from build123d import *

# Parameters (mm, degrees)
SKETCH_1_W                   = 110
SKETCH_1_H                   = 110
EXTRUDE_1_DEPTH              = 110
SKETCH_2_W                   = 100
SKETCH_2_H                   = 100
CUT_EXTRUDE_1_DEPTH          = 105
SKETCH_3_W                   = 13.484754144
SKETCH_3_H                   = 100
CUT_EXTRUDE_2_DEPTH          = 105
HOLE_WIZARD_M4_6_D           = 3.3
HOLE_WIZARD_M4_6_CSINK_D     = 4.05
HOLE_WIZARD_M4_6_CSINK_ANGLE = 90
HOLE_WIZARD_M4_7_D           = 3.3
HOLE_WIZARD_M4_7_CSINK_D     = 4.05
HOLE_WIZARD_M4_7_CSINK_ANGLE = 90
PATTERN_CIRCULAR_2_COUNT     = 6


# Read off the part's stored shape, not the designer's step: 阵列(圆周)1
with BuildPart() as part:
    # 草图1 → 凸台-拉伸1 (new body)
    with BuildSketch(Plane(origin=(0, 0, 0), x_dir=(1, 0, 0), z_dir=(0, 1, 0))):
        Rectangle(SKETCH_1_W, SKETCH_1_H)
    extrude(amount=EXTRUDE_1_DEPTH)

    # 草图2 → 切除-拉伸1 (cut)
    with BuildSketch(Plane(origin=(0, 110, 0), x_dir=(1, 0, 0), z_dir=(0, 1, 0))):
        Rectangle(SKETCH_2_W, SKETCH_2_H)
    extrude(amount=-CUT_EXTRUDE_1_DEPTH, mode=Mode.SUBTRACT)

    # 草图3 → 切除-拉伸2 (cut)
    with BuildSketch(Plane(origin=(0, 110, 0), x_dir=(1, 0, 0), z_dir=(0, 1, 0))):
        with Locations((56.742377072, 0)):
            Rectangle(SKETCH_3_W, SKETCH_3_H)
    extrude(amount=-CUT_EXTRUDE_2_DEPTH, mode=Mode.SUBTRACT)

    # M4 螺纹孔6 (through all)
    with Locations(Plane.XZ):
        with Locations((0, 17.25)):
            CounterSinkHole(HOLE_WIZARD_M4_6_D / 2, HOLE_WIZARD_M4_6_CSINK_D / 2, counter_sink_angle=HOLE_WIZARD_M4_6_CSINK_ANGLE)

    # 阵列(圆周)1 outline → 阵列(圆周)1 (revolve, cut)
    with BuildSketch(Plane(origin=(-14.954860189, 0, 8.615807444), x_dir=(1, 0, 0), z_dir=(0, 0, 1))):
        Polygon((1.65, 0.375), (1.65, 5), (0, 5), (0, 0), (2.025, 0), align=None)
    revolve(axis=Axis((-14.954860189, 0, 8.615807444), (0, 1, 0)), mode=Mode.SUBTRACT)

    # Pattern Circular 1 2 outline → Pattern Circular 1 2 (revolve, cut)
    with BuildSketch(Plane(origin=(-14.954860189, 0, -8.652577668), x_dir=(1, 0, 0), z_dir=(0, 0, 1))):
        Polygon((1.65, 0.375), (1.65, 5), (0, 5), (0, 0), (2.025, 0), align=None)
    revolve(axis=Axis((-14.954860189, 0, -8.652577668), (0, 1, 0)), mode=Mode.SUBTRACT)

    # Pattern Circular 1 3 outline → Pattern Circular 1 3 (revolve, cut)
    with BuildSketch(Plane.XY.offset(-17.286770224)):
        Polygon((1.65, 0.375), (1.65, 5), (0, 5), (0, 0), (2.025, 0), align=None)
    revolve(axis=Axis((0, 0, -17.286770224), (0, 1, 0)), mode=Mode.SUBTRACT)

    # Pattern Circular 1 4 outline → Pattern Circular 1 4 (revolve, cut)
    with BuildSketch(Plane(origin=(14.954860189, 0, -8.652577668), x_dir=(1, 0, 0), z_dir=(0, 0, 1))):
        Polygon((1.65, 0.375), (1.65, 5), (0, 5), (0, 0), (2.025, 0), align=None)
    revolve(axis=Axis((14.954860189, 0, -8.652577668), (0, 1, 0)), mode=Mode.SUBTRACT)

    # Pattern Circular 1 5 outline → Pattern Circular 1 5 (revolve, cut)
    with BuildSketch(Plane(origin=(14.954860189, 0, 8.615807444), x_dir=(1, 0, 0), z_dir=(0, 0, 1))):
        Polygon((1.65, 0.375), (1.65, 5), (0, 5), (0, 0), (2.025, 0), align=None)
    revolve(axis=Axis((14.954860189, 0, 8.615807444), (0, 1, 0)), mode=Mode.SUBTRACT)

    # M4 螺纹孔7 (through all)
    with Locations(Plane(origin=(-50, 0, 0), x_dir=(0, 0, -1), z_dir=(1, 0, 0))):
        with Locations((0, 74.75)):
            hole_wizard_m4_7 = CounterSinkHole(HOLE_WIZARD_M4_7_D / 2, HOLE_WIZARD_M4_7_CSINK_D / 2, counter_sink_angle=HOLE_WIZARD_M4_7_CSINK_ANGLE)

    # 阵列(圆周)2: M4 螺纹孔7 ×6 about axis
    pattern_circular_2_axis = Axis((0, 57.478809906, 0), (1, 0, 0))
    for i in range(1, PATTERN_CIRCULAR_2_COUNT):
        add(hole_wizard_m4_7.rotate(pattern_circular_2_axis, i * 360 / PATTERN_CIRCULAR_2_COUNT), mode=Mode.SUBTRACT)


solid = part.part
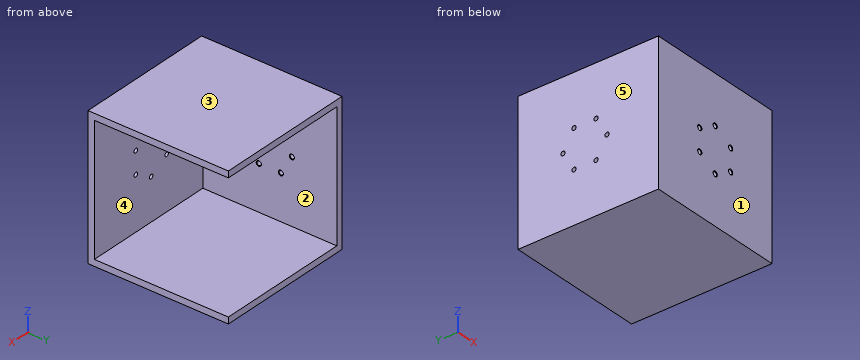
Can you work these out from the model? Positions are in its coordinate system, mm. Face numbers are marked on the shaded views. A direction names the side the tool comes from. Give positions to 0.01 mm unless a question says otherwise; leave off trailing zeros. Order: outer loops, then holes, each group sorted by start corner. A loop starts at its lowest first (then second) coordinate and runs counter-clockwise, first axis right, second up. Notation, with made-up numbers: M -7,62.25 L 36,62.25 A15 cw 36,79.25 Z; hole C -10,-2.5 d11. An arc over 180 degrees is marked long. One line per item, written item: value.
Item 1: If we mould it in two halves opening along Z, with no side actions, what happens to the marked faces 1, 2 and 3? For each: pulls with the +Z half, pulls with the -Z half, needs draft (parallel to the pull), parting line crosses it, or undercut.
Verdict:
face 1: needs draft
face 2: undercut
face 3: pulls with the +Z half
Item 2: Please list where these lines run through material, in increasing order: line 1 (Z direction, x = 0, y = 2); line 2 (Z direction, x = -35.5, y = 19.5); line 3 (Y direction, x = -14, z = -15.5).
Verdict:
line 1: -55 to -18.94, -15.64 to 15.6, 18.9 to 55
line 2: -55 to -50, 50 to 55
line 3: 0 to 5
Item 3: If we section it at C-C on x = 0: Write out the boundary of the cut face in (y, z) (3 decimals).
Verdict:
outline: M 0,-55 L 110,-55 L 110,-50 L 5,-50 L 5,-18.937 L 0.375,-18.937 L 0,-19.312 Z; M 0,-15.262 L 0.375,-15.637 L 5,-15.637 L 5,15.6 L 0.375,15.6 L 0,15.225 Z; M 0,19.275 L 0.375,18.9 L 5,18.9 L 5,50 L 110,50 L 110,55 L 0,55 Z
Item 4: For pin 1 (10 mm diameter, centred on x = -4, z = 25, fed in from +Y); pin 2 (5 mm diameter, centred on y = 47.5, z = -13, fed in from +X), each with a flat end and sliding along its axis, tell me the tip position at first contact or that it passes through.
Verdict:
pin 1: y = 5
pin 2: x = -50
Item 5: If we section it at B-B on y = 74.75: Write out the boundary of the cut face in (x, z) (3 decimals), and give its area (3 significant figures).
Verdict:
outline: M -55,-55 L 55,-55 L 55,-50 L -50,-50 L -50,-2.025 L -50.375,-1.65 L -55,-1.65 Z; M -55,1.65 L -50.375,1.65 L -50,2.025 L -50,50 L 55,50 L 55,55 L -55,55 Z
area: 1,580 mm2
Item 6: For the marked faces 4 and 5, which set-ups out of +Z, -Z, +X, -X, +Y, -Y let a thin tool reach every point of the face, with its end or its side?
Verdict:
face 4: +X, +Y
face 5: +Z, -Z, -X, +Y, -Y
Item 7: If we section it at D-D on y = 20: Write out the boundary of the cut face in (x, z).
Verdict:
outline: M -55,-55 L 55,-55 L 55,-50 L -50,-50 L -50,50 L 55,50 L 55,55 L -55,55 Z
Item 8: If we section it at A-A on z = 0: Write out the boundary of the cut face in (x, y) (3 decimals).
Verdict:
outline: M -55,0 L 55,0 L 55,5 L -50,5 L -50,38.183 L -50.375,38.558 L -55,38.558 Z; M -55,41.858 L -50.375,41.858 L -50,42.233 L -50,72.725 L -50.375,73.1 L -55,73.1 Z; M -55,76.4 L -50.375,76.4 L -50,76.775 L -50,110 L -55,110 Z
